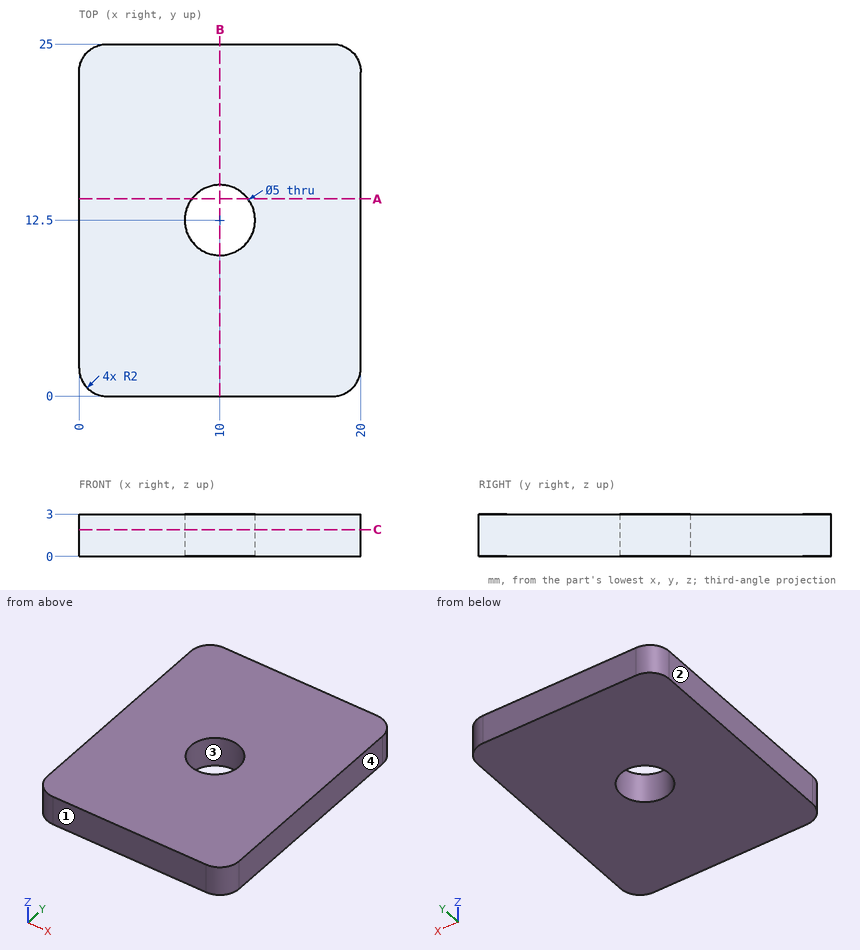
For this review, use the dimensioned drawing (mm, ordinates from the lowest corner) and the shaded views. Give positions to 0.01 mm unless a question says otherwise; leave off trailing zeros. Order: outer loops, then holes, each group sorted by start corner. A loop starts at its lowest first (then second) coordinate and runs counter-clockwise, first axis right, second up. Notation, with made-up numbers: M -10.5,-21 L 0.5,-21 A30 ccw 0.5,17 Z; hole C 32.25,-32.5 d10. An arc over 180 degrees is marked long. Use one line per item in the form item = value. Start each with the question number.
Item 1: We need section C-C on z = 1.9. Give the boundary of the cut face in (x, y).
Item 2: We need section A-A on y = 14. Give the boundary of the cut face in (x, z), plus the area to 3 significant figures.
Item 3: We need section B-B on x = 10. Give the boundary of the cut face in (y, z), plus the area to 3 significant figures.
Item 4: To check wall thickness, follow line 1 along Y through (x, z) = (10, 0.7); line 2 along X through (y, z) = (14.75, 2.9); line 3 along Y through (x, z) = (12, 0.7). State the ranges of each line that lie inside material, in increasing order. Write a range as from..to.
Item 5: The part is to be moulded in two halves that separate along X. For the marked faces 1, 2, 3 and 4, say which applies: pulls with the +X half, pulls with the -X half, needs draft (parallel to the pull), parting line crosses it, or undercut.
Completed:
q1.outline = M 0,2 A2 ccw 2,0 L 18,0 A2 ccw 20,2 L 20,23 A2 ccw 18,25 L 2,25 A2 ccw 0,23 Z; hole C 10,12.5 d5
q2.outline = M 0,0 L 8,0 L 8,3 L 0,3 Z; M 12,0 L 20,0 L 20,3 L 12,3 Z
q2.area = 48.0 mm²
q3.outline = M 0,0 L 10,0 L 10,3 L 0,3 Z; M 15,0 L 25,0 L 25,3 L 15,3 Z
q3.area = 60.0 mm²
q4.line_1 = 0..10, 15..25
q4.line_2 = 0..8.91, 11.09..20
q4.line_3 = 0..11, 14..25
q5.face_1 = needs draft
q5.face_2 = pulls with the -X half
q5.face_3 = undercut
q5.face_4 = pulls with the +X half
